```python
from build123d import *

# Parameters (mm, degrees)
F1_DEPTH  = 18
F3_DEPTH  = 5
F5_DEPTH  = 7
F6_R      = 12.5
F6_R_2    = 3.5
F7_DEPTH  = 25
F8_R      = 10
F8_R_2    = 3.5
F9_DEPTH  = 1
F10_R     = 3.902724
F11_DEPTH = 25
F12_R     = 10
F12_R_2   = 3.902724
F13_DEPTH = 1


with BuildPart() as f1:
    # F0 (on Top) → F1 (new body)
    with BuildSketch(Plane.XY):
        with BuildLine():
            Line((600, 60), (600, 0))
            Line((600, 0), (1200, 0))
            Line((1200, 0), (1200, 350))
            Line((1200, 350), (0, 350))
            Line((0, 350), (0, 90))
            Line((0, 90), (570, 90))
            ThreePointArc((570, 90), (591.213203, 81.213203), (600, 60))
        make_face()
    extrude(amount=F1_DEPTH)

    # F2 (on face) → F3 (join)
    with BuildSketch(Plane(origin=(0, 0, 0), x_dir=(1, 0, 0), z_dir=(0, 0, -1))):
        with BuildLine():
            Line((600, 0), (600, -60))
            ThreePointArc((600, -60), (591.213203, -81.213203), (570, -90))
            Line((570, -90), (0, -90))
            Line((0, -90), (0, -350))
            Line((0, -350), (1200, -350))
            Line((1200, -350), (1200, 0))
            Line((1200, 0), (600, 0))
        make_face()
        with BuildLine():
            Line((369, -105), (555, -105))
            ThreePointArc((555, -105), (558.535534, -106.464466), (560, -110))
            Line((560, -110), (560, -150))
            ThreePointArc((560, -150), (558.535534, -153.535534), (555, -155))
            Line((555, -155), (369, -155))
            ThreePointArc((369, -155), (365.464466, -153.535534), (364, -150))
            Line((364, -150), (364, -110))
            ThreePointArc((364, -110), (365.464466, -106.464466), (369, -105))
        make_face(mode=Mode.SUBTRACT)
    extrude(amount=F3_DEPTH)

    # F4 (on face) → F5 (cut)
    with BuildSketch(Plane(origin=(0, 0, -5), x_dir=(1, 0, 0), z_dir=(0, 0, -1))):
        with BuildLine():
            Line((125, -90), (0, -90))
            Line((0, -90), (0, -114.8))
            Line((0, -114.8), (120, -114.8))
            ThreePointArc((120, -114.8), (123.535534, -113.335534), (125, -109.8))
            Line((125, -109.8), (125, -90))
        make_face()
    extrude(amount=-F5_DEPTH, mode=Mode.SUBTRACT)

    # F6 (on face) → F7 (cut)
    with BuildSketch(Plane(origin=(0, 0, 0), x_dir=(1, 0, 0), z_dir=(0, 0, -1))):
        with Locations((525, -130)):
            Circle(F6_R)
        with Locations((399, -130)):
            Circle(F6_R)
        with Locations((371, -112)):
            Circle(F6_R_2)
        with Locations((427, -112)):
            Circle(F6_R_2)
        with Locations((371, -148)):
            Circle(F6_R_2)
        with Locations((427, -148)):
            Circle(F6_R_2)
        with Locations((497, -148)):
            Circle(F6_R_2)
        with Locations((497, -112)):
            Circle(F6_R_2)
        with Locations((553, -112)):
            Circle(F6_R_2)
        with Locations((553, -148)):
            Circle(F6_R_2)
    extrude(amount=-F7_DEPTH, mode=Mode.SUBTRACT)

    # F8 (on face) → F9 (cut)
    with BuildSketch(Plane.XY.offset(18)):
        with Locations((371, 148)):
            Circle(F8_R)
        with Locations((371, 148)):
            Circle(F8_R_2, mode=Mode.SUBTRACT)
        with Locations((427, 148)):
            Circle(F8_R)
        with Locations((427, 148)):
            Circle(F8_R_2, mode=Mode.SUBTRACT)
        with Locations((497, 148)):
            Circle(F8_R)
        with Locations((497, 148)):
            Circle(F8_R_2, mode=Mode.SUBTRACT)
        with Locations((553, 148)):
            Circle(F8_R)
        with Locations((553, 148)):
            Circle(F8_R_2, mode=Mode.SUBTRACT)
        with Locations((553, 112)):
            Circle(F8_R)
        with Locations((553, 112)):
            Circle(F8_R_2, mode=Mode.SUBTRACT)
        with Locations((497, 112)):
            Circle(F8_R)
        with Locations((497, 112)):
            Circle(F8_R_2, mode=Mode.SUBTRACT)
        with Locations((427, 112)):
            Circle(F8_R)
        with Locations((427, 112)):
            Circle(F8_R_2, mode=Mode.SUBTRACT)
        with Locations((371, 112)):
            Circle(F8_R)
        with Locations((371, 112)):
            Circle(F8_R_2, mode=Mode.SUBTRACT)
    extrude(amount=-F9_DEPTH, mode=Mode.SUBTRACT)

    # F10 (on face) → F11 (cut)
    with BuildSketch(Plane(origin=(0, 0, 2), x_dir=(1, 0, 0), z_dir=(0, 0, -1))):
        with Locations((111.9, -103.2)):
            Circle(F10_R)
        with Locations((91.9, -103.2)):
            Circle(F10_R)
        with Locations((71.9, -103.2)):
            Circle(F10_R)
        with Locations((51.9, -103.2)):
            Circle(F10_R)
        with Locations((31.9, -103.2)):
            Circle(F10_R)
    extrude(amount=-F11_DEPTH, mode=Mode.SUBTRACT)

    # F12 (on face) → F13 (cut)
    with BuildSketch(Plane.XY.offset(18)):
        with Locations((31.9, 103.2)):
            Circle(F12_R)
        with Locations((31.9, 103.2)):
            Circle(F12_R_2, mode=Mode.SUBTRACT)
        with Locations((71.9, 103.2)):
            Circle(F12_R)
        with Locations((71.9, 103.2)):
            Circle(F12_R_2, mode=Mode.SUBTRACT)
        with Locations((111.9, 103.2)):
            Circle(F12_R)
        with Locations((111.9, 103.2)):
            Circle(F12_R_2, mode=Mode.SUBTRACT)
    extrude(amount=-F13_DEPTH, mode=Mode.SUBTRACT)


solid = f1.part
```
CAD build for the part. Positions are in the model's coordinates, mm. A direction names the side the tool comes from. Give positions to 0.01 mm unless a question says otherwise; leave off trailing zeros. Order: outer loops, then holes, each group sorted by start corner. A loop starts at its lowest first (then second) coordinate and runs counter-clockwise, first axis right, second up.
(1) Saw through at B-B, the plane x = 327.5. Give the cut face in (y, z).
(2) Drill centre lines: L1, parallel to Y at x = 427, z = 17.4; L2, parallel to X at y = 112, z = 4; L3, parallel to X at y = 130, z = 9. Where is each one in solid material? Low to high.
(3) Tool access for faces 1 (the cylindrical face through (405.72, 119.46, 8.87)), 2 (the flat face through (371, 108, 17)): list every direction of +Z, -Z, +X, -X, +Y, -Y with a clear straight run to the whole face (end or side of a thin tool).
(4) Flat gauge pins, fed straight in: pin 1 (18 mm diameter, centred on x = 31.9, y = 103.2, fed in from -Z); pin 2 (6 mm diameter, centred on y = 116, z = -1, fed in from -X); pin 3 (16 mm diameter, centred on x = 551.5, y = 112.5, fed in from +Z); pin 4 (10 mm diameter, centred on y = 40, z = 8, fed in from -X). Where does each tip first touch, or does it go through?
(5) Saw through at A-A, the plane y = 41.5. Give the cut face in (x, z).
(6) Mould opens along Y. For faces 3 (the flat face through (600, 30, 7)), 4 (the flat face through (592, 350, 7)), 5 (the flat face through (557, 112, 17)) say: released by +Y, released by -Y, zero draft, split by the parting line, or undercut.
Results found:
1. outline: (90, -5) - (350, -5) - (350, 18) - (90, 18) - close
2. L1: y = 90 to 102, 122 to 138, 158 to 350
2. L2: x = 0 to 367.5, 374.5 to 423.5, 430.5 to 493.5, 500.5 to 549.5, 556.5 to 1200
2. L3: x = 0 to 386.5, 411.5 to 512.5, 537.5 to 1200
3. face 1: +Z, -Z
3. face 2: +Z
4. pin 1: stops at z = 2
4. pin 2: stops at x = 0
4. pin 3: stops at z = 17
4. pin 4: stops at x = 600
5. outline: (600, -5) - (1200, -5) - (1200, 18) - (600, 18) - close
6. face 3: zero draft
6. face 4: released by +Y
6. face 5: undercut
